Work out the finished part from the listing and answer in its coordinate system (mm). Face numbers are marked on the shaded views. Coordinates: 2 decimals unless noted, no trailing zeros. Write each loop counter-clockwise with the first axis right and the second up, starting at its lowest first coordinate (ties: lowest second). Pieces come first, ordered by that corner, then holes. Notation, with made-up numbers: M -28,78.25 L 14,78.25 A26 ccw 14,115.25 Z; hole C 71.5,-28.5 d4. An arc over 180 degrees is marked long. Use CSV: the item, a comma, the result in double quotes.
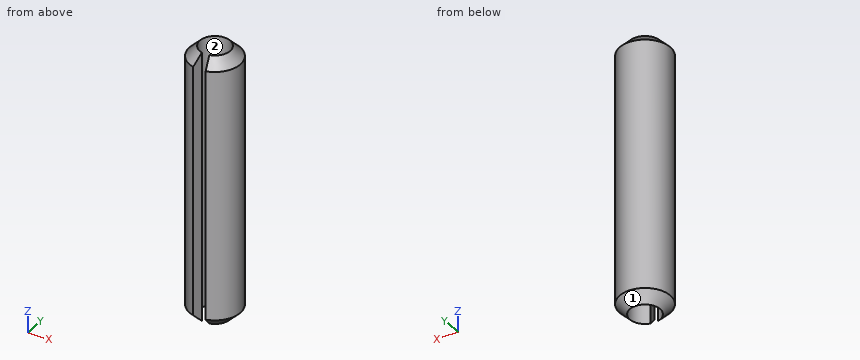
from build123d import *

# Parameters (mm, degrees)
BASE_EXTRUSION_DEPTH = 16
CHANFREIN1_SIZE      = 0.6


with BuildPart() as part:
    # Esquisse1 → Base-Extrusion (new body)
    with BuildSketch(Plane.XY):
        with BuildLine():
            Line((-0.222603523, -0.872036508), (-0.371005872, -1.45339418))
            ThreePointArc((-0.371005872, -1.45339418), (0, 1.5), (0.371005872, -1.45339418))
            Line((0.371005872, -1.45339418), (0.222603523, -0.872036508))
            ThreePointArc((0.222603523, -0.872036508), (0, 0.9), (-0.222603523, -0.872036508))
        make_face()
    extrude(amount=-BASE_EXTRUSION_DEPTH)

    # Chanfrein1
    chanfrein1_edges = [part.edges().sort_by_distance(p)[0] for p in [
        (0, 1.5, 0),
        (0, 1.5, -16),
    ]]
    chamfer(chanfrein1_edges, length=CHANFREIN1_SIZE - 0.0001)  # a hair under: the kernel refuses the full size


solid = part.part
Item 1: Consider probe 1 along X at (y, z) = (0, -9); probe 2 along X at (y, z) = (-1.1, -6.25); probe 3 along Y at (x, z) = (0, -5.5). Determine where each line is inside the solid, lowest interval first.
Answer:
probe 1,"x = -1.5 to -0.9, 0.9 to 1.5"
probe 2,"x = -1.02 to -0.28, 0.28 to 1.02"
probe 3,"y = 0.9 to 1.5"
Item 2: For a pull along X with two mould halves and no side action, classify the marked faces 1 and 2 as released by +X, released by -X, zero draft, split by the parting line, or undercut.
Answer:
face 1,"split by the parting line"
face 2,"undercut"
Item 3: The part is cut by section B-B (z = -3). Write down the section's boundary in (x, y), then the cut area to 3 significant figures.
Answer:
outline,"M -0.37,-1.45 L -0.22,-0.87 A0.9 cw long 0.22,-0.87 L 0.37,-1.45 A1.5 ccw long Z"
area,"4.16 mm2"
Item 4: Given pin 1 (1.5 mm diameter, centred on x = 0.5, y = 0, fed in from +Z), flat-ended and moving along its own axis, determine where the tip first touches the part or whether it passes through.
Answer:
pin 1,"stops at z = 0"
